Verification items for this drawing (mm, ordinates from the low corner). A direction names the side the tool comes from. Give positions to 0.01 mm unless a question says otherwise; leave off trailing zeros. Loops run counter-clockwise (first coordinate to the right, second up) from the corner with the lowest first, then second, coordinate; pieces in that order, holes last. Notation, with made-up numbers: (-13.75, 35) -> (29.25, 35) arc R32 ccw to (29.25, 74) -> close; hole circle Ø9 at (43, -19). An arc over 180 degrees is marked (long way). Write each question's results on one line, items separated by ' | '. Start each with the question number.
Item 1: Scan lines: line 1 along X through (y, z) = (13.5, 72); line 2 along X through (y, z) = (45.5, 34.5); line 3 along Z through (x, y) = (26, 47). Record each from-to range of solid material in increasing order.
Item 2: Cross-section at D-D on x = 28.5. Enter the section's corners in (y, z), then the cut area to 3 significant figures.
Item 3: Cross-section at A-A on z = 50.8. Enter the section's corners in (x, y), then the cut area to 3 significant figures.
Item 4: Access from +Z, -Z, +X, -X, +Y, -Y to the whole of each face (thin tool, end or side, straight path). Record for the marked faces 1, 2 and 3.
Item 5: Gauge pin test, flat ends, axial feed: pin 1 Ø10 at (y, z) = (57, 25) entering from +X; pin 2 Ø1.5 at (x, z) = (94, 17) entering from -Y; pin 3 Ø6 at (x, z) = (124, 43) entering from -Y. Record the tip position at first contact, or that the pin passes through.
Item 6: Cross-section at C-C on x = 267. Enter the section's corners in (y, z).
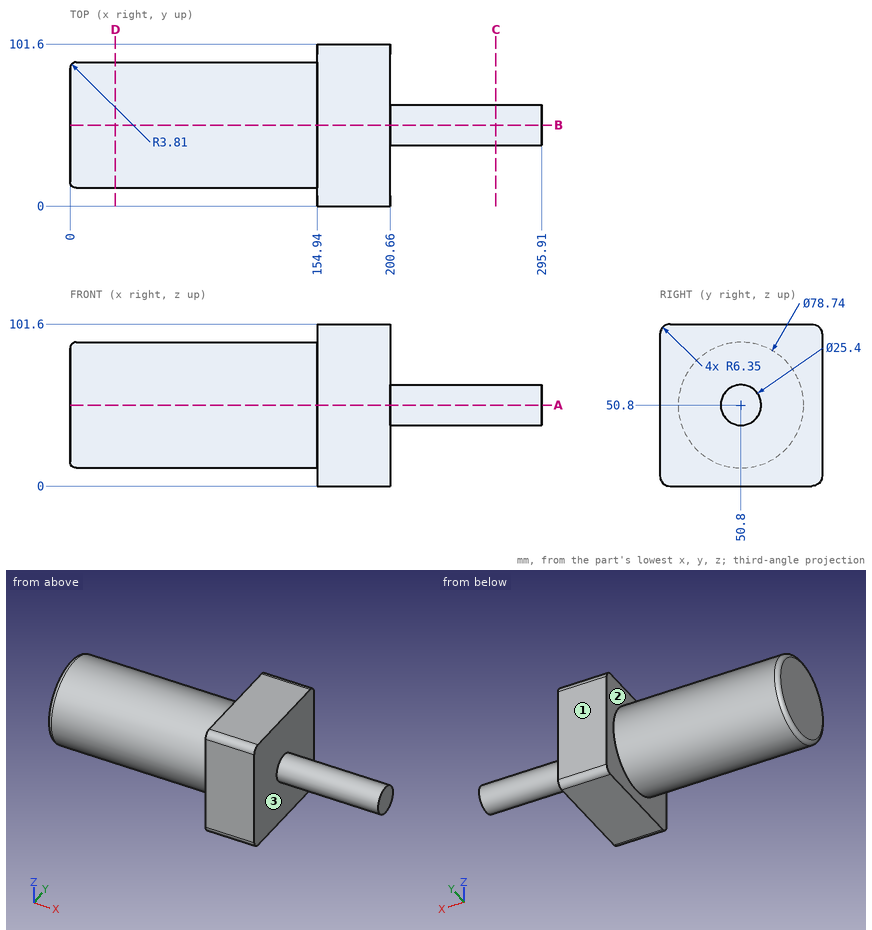
Answer sheet:
1) line 1: x = 154.94 to 200.66 | line 2: x = 0 to 200.66 | line 3: z = 11.61 to 89.99
2) outline: circle Ø78.74 at (50.8, 50.8) | area: 4,870 mm²
3) outline: (0, 15.24) arc R3.81 ccw to (3.81, 11.43) -> (154.94, 11.43) -> (154.94, 0) -> (200.66, 0) -> (200.66, 38.1) -> (295.91, 38.1) -> (295.91, 63.5) -> (200.66, 63.5) -> (200.66, 101.6) -> (154.94, 101.6) -> (154.94, 90.17) -> (3.81, 90.17) arc R3.81 ccw to (0, 86.36) -> close | area: 19,300 mm²
4) face 1: +Z, -Z, +X, -X, +Y | face 2: -X | face 3: +X
5) pin 1: stops at x = 200.66 | pin 2: stops at y = 29.41 | pin 3: stops at y = 11.72
6) outline: circle Ø25.4 at (50.8, 50.8)
